Drawing for the job (mm, zero at the part's lowest x, y, z). A direction names the side the tool comes from. Give positions to 0.01 mm unless a question says otherwise; leave off trailing zeros. Write each loop counter-clockwise with the first axis right and the second up, starting at its lowest first coordinate (ties: lowest second). Pieces come first, ordered by that corner, then holes. Notation, with made-up numbers: M 5,52 L 63,52 A27 ccw 63,83 Z; hole C 86.25,62.25 d3. An arc over 180 degrees is marked long. Use CSV: the item, a comma, the result in double quotes. Start each with the question number.
1. 3-axis set-ups, long thin cutter, end or side, ignore diameter. For the marked faces 4, 5 and 6: which of +Z, -Z, +X, -X, +Y, -Y reach the whole face in a straight line?
2. Band-saw the part on B-B, the plane x = 35. List the corners of the cut face in (y, z).
3. Drop flat-ended pins along their axis: pin 1 Ø1.5 at (y, z) = (5.5, 7.5) entering from +X; pin 2 Ø3 at (x, y) = (35, 5.048) entering from +Z; pin 3 Ø0.9 at (y, z) = (5.5, 7.5) entering from -X. Give the stop position or say it passes through.
4. Band-saw the part on D-D, the plane z = 2.25. List the corners of the cut face in (x, y).
5. Drill centre lines: line 1 along Y through (x, z) = (35, 4.1); line 2 along X through (y, z) = (4, 2.5); line 3 along X through (y, z) = (4.75, 7.25). Where is each one in solid material? Low to high. Write a range as from..to.
6. Mould opens along Y. For the marked faces 1, 2 and 3 say: pulls with the +Y half, pulls with the -Y half, needs draft (parallel to the pull), parting line crosses it, or undercut.
7. Band-saw the part on C-C, the plane y = 7.75. List the corners of the cut face in (x, z), then the cut area to 4 significant figures.
8. Band-saw the part on A-A, the plane y = 5.75. List the corners of the cut face in (x, z), then the cut area to 3 significant figures.
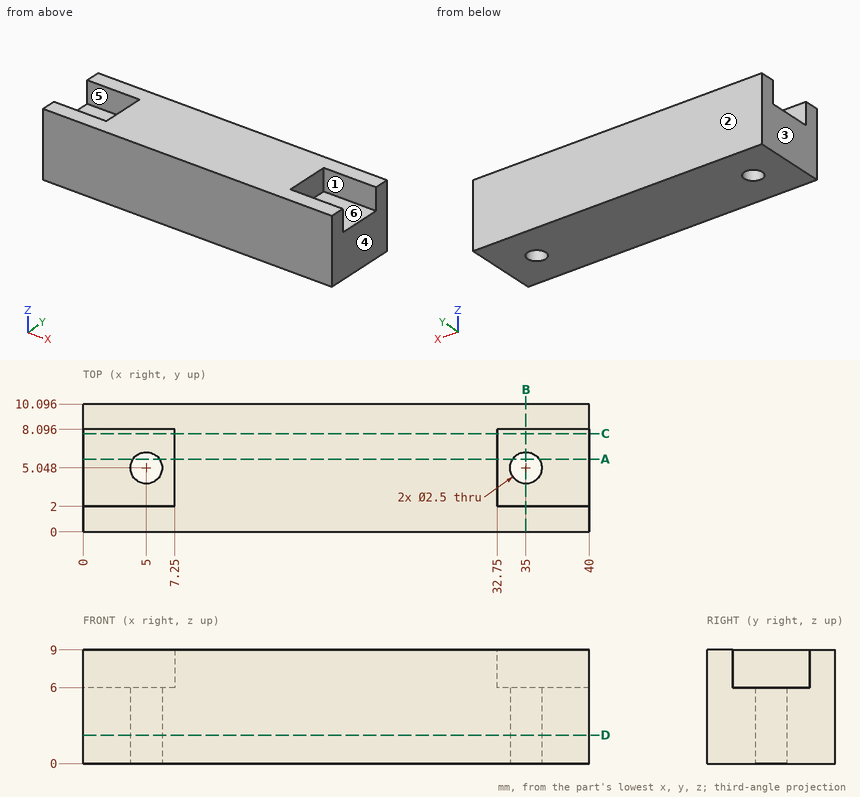
Output:
1,face 4,"+Z, -Z, +X, +Y, -Y"
1,face 5,"+Z, -X"
1,face 6,"+Z, +X"
2,outline,"M 0,0 L 3.8,0 L 3.8,6 L 2,6 L 2,9 L 0,9 Z; M 6.3,0 L 10.1,0 L 10.1,9 L 8.1,9 L 8.1,6 L 6.3,6 Z"
3,pin 1,"stops at x = 32.75"
3,pin 2,"stops at z = 6"
3,pin 3,"stops at x = 7.25"
4,outline,"M 0,0 L 40,0 L 40,10.1 L 0,10.1 Z; hole C 5,5.05 d2.5; hole C 35,5.05 d2.5"
5,line 1,"y = 0..3.8, 6.3..10.1"
5,line 2,"x = 0..4.32, 5.68..34.32, 35.68..40"
5,line 3,"x = 7.25..32.75"
6,face 1,"undercut"
6,face 2,"pulls with the +Y half"
6,face 3,"needs draft"
7,outline,"M 0,0 L 40,0 L 40,6 L 32.75,6 L 32.75,9 L 7.25,9 L 7.25,6 L 0,6 Z"
7,area,"316.5 mm²"
8,outline,"M 0,0 L 3.97,0 L 3.97,6 L 0,6 Z; M 6.03,0 L 33.97,0 L 33.97,6 L 32.75,6 L 32.75,9 L 7.25,9 L 7.25,6 L 6.03,6 Z; M 36.03,0 L 40,0 L 40,6 L 36.03,6 Z"
8,area,"292 mm²"
